For this review, take the finished solid that the model builds, in its own axes (mm). A direction names the side the tool comes from. Give positions to 0.01 mm unless a question says otherwise; leave off trailing zeros. Loops run counter-clockwise (first coordinate to the right, second up) from the corner with the lowest first, then second, coordinate; pieces in that order, holes last. Notation, with made-up numbers: (42, 71.5) - (85, 71.5) arc R14 ccw to (85, 79.5) - close; hole circle Ø10 at (88.5, 31.5). An arc over 180 degrees is marked (long way). Answer in a Markdown table with one row per item.
Autodesk Inventor part; units mm, degrees
ref_plane "YZ Plane" through (0, 0, 0) normal (1, 0, 0) x (0, 1, 0)
ref_plane "XZ Plane" through (0, 0, 0) normal (0, 1, 0) x (-1, 0, 0)
ref_plane "XY Plane" through (0, 0, 0) normal (0, 0, 1) x (1, 0, 0)
sketch "Boceto1" plane through (0, 0, 0) normal (0, 0, 1) x (1, 0, 0)
  line L0 (-17.5, 10) -> (17.5, 10)
  line L1 (17.5, 10) -> (17.5, -10)
  line L2 (17.5, -10) -> (-17.5, -10)
  line L3 (-17.5, -10) -> (-17.5, 10)
  line L4 (0, 0) -> (0, 1.7227)
  line L5 (0, 0) -> (-2.1619, 0)
  line L6 (17.5, -10) -> (-0.5, -10)
  line L7 (-0.5, -10) -> (-0.5, -27)
  line L8 (-0.5, -27) -> (17.5, -27)
  line L9 (17.5, -27) -> (17.5, -10)
  circle A0 centre (12.5, 0) radius 2
  circle A1 centre (-12.5, 0) radius 2
  point P0 (-0.5, -10)
  dimension "d14" = 35
  dimension "d15" = 20
  dimension "d16" = 18
  dimension "d17" = 17
  dimension "d18" = 4
  dimension "d19" = 4
  dimension "d20" = 5
  dimension "d21" = 5
extrude "Extrusión1" add sketch "Boceto1" along normal blind 10
sketch "Boceto2" plane through (-0.5, -27, 0) normal (0, -1, 0) x (1, 0, 0)
  line L0 (18, 10) -> (-17, 10)
  line L1 (18, 10) -> (-2, 10)
  line L2 (-2, 10) -> (-2, -20)
  line L3 (-2, -20) -> (18, -20)
  line L4 (18, -20) -> (18, 10)
  point P0 (0.5, 0)
  point P1 (-2, 10)
  dimension "d22" = 30
  dimension "d53" = 20
extrude "Extrusión2" add sketch "Boceto2" along normal blind 5
sketch "Boceto4" plane through (-17.5, -10, 0) normal (-1, 0, 0) x (0, 0, 1)
  line L0 (0, 0) -> (0, -17)
  line L1 (10, 20) -> (10, 0)
  line L2 (10, 0) -> (-20, 0)
  line L3 (-20, 0) -> (-20, -5)
  line L4 (-20, -5) -> (10, -5)
  line L5 (10, -5) -> (10, 0)
  line L6 (10, -22) -> (-20, -22)
  point P0 (0, 10)
  dimension "d32" = 5
  dimension "d43" = 30
  dimension "d44" = 30
extrude "Extrusión4" add sketch "Boceto4" against normal up to surface (35 mm away)
sketch "Boceto5" plane through (-0.5, -32, 0) normal (0, -1, 0) x (1, 0, 0)
  circle A0 centre (8, -9) radius 1.75
  line L0 (18, -20) -> (18, 10)
  circle A1 centre (-12, -9) radius 1.75
  line L1 (-2, -20) -> (18, -20)
  line L2 (-17, -20) -> (18, -20)
  line L3 (-17, -20) -> (-17, 10)
  line L4 (-17, 0) -> (18, 0)
  point P0 (0.5, 0)
  point P1 (0, 0)
  dimension "d33" = 3.5
  dimension "d34" = 10
  dimension "d37" = 3.5
  dimension "d38" = 5
  dimension "d41" = 9
  dimension "d42" = 9
extrude "Extrusión5" cut sketch "Boceto5" against normal up to surface (22 mm away) contours A0 | A1
sketch "Boceto7" plane through (17.5, -27, -20) normal (0, 0, -1) x (-1, 0, 0)
  line L0 (0, -5) -> (20, -5)
  line L1 (35, 17) -> (0, 17)
  line L2 (10, -5) -> (10, -5.3641)
  line L3 (13.5, -5) -> (13.5, 17)
  line L4 (6.5, -5) -> (6.5, 17)
  point P0 (17.5, 27)
  dimension "d47" = 7
extrude "Extrusión7" add sketch "Boceto7" along normal blind 5
equation "\"d19\" = d18"
equation "\"d20\" = d21"
equation "\"d44\" = d43"
equation "\"d37\" = d33"
properties part number "Soporte Idler Z" material "Hormigón reforzado con fibra de vidrio"
1. We need section D-D, the plane z = -18. Give the boundary of the cut face in (x, y), and give its area (3 significant figures).
Values:
| item | result |
|---|---|
| outline | (-17.5, -15) - (17.5, -15) - (17.5, -10) - (-17.5, -10) - close; (-2.5, -32) - (17.5, -32) - (17.5, -27) - (-2.5, -27) - close |
| area | 275 mm^2 |
2. Mouldability with a two-part tool opening along Z and no side actions: class faces 6 (the face through (-2.5, -29, -5)), 7 (the face through (14, -29, -20)), 8 (the face through (8.4, -29.5, -7.5)) as released by +Z, released by -Z, zero draft, split by the parting line, or undercut.
Values:
| item | result |
|---|---|
| face 6 | zero draft |
| face 7 | released by -Z |
| face 8 | undercut |
3. Clearance check with flat-ended pins moving along their axes: pin 1 (2.5 mm diameter, centred on x = 15.5, y = -29, fed in from -Z); pin 2 (4 mm diameter, centred on y = -25.5, z = -4, fed in from -X); pin 3 (1.5 mm diameter, centred on y = -21, z = -23, fed in from -X); pin 4 (12 mm diameter, centred on y = -6.5, z = -2.5, fed in from +X). State where each tip first meets the part, or that it passes through.
Values:
| item | result |
|---|---|
| pin 1 | stops at z = -20 |
| pin 2 | stops at x = -2.5 |
| pin 3 | stops at x = 4 |
| pin 4 | stops at x = 17.5 |
4. For faces 1 (the face through (8, -21, 0)), 2 (the face through (14, -12, -20)), 3 (the face through (0, 0, 0)), 4 (the face through (-0.5, -21, 5)), 5 (the face through (4, -21, -22)), list the 3-axis set-ups (+Z, -Z, +X, -X, +Y, -Y) from which the entire face can be reached by the end or side of a thin tool; tool diameter is ignored.
Values:
| item | result |
|---|---|
| face 1 | +X, -X |
| face 2 | -Z, +X, +Y, -Y |
| face 3 | -Z, +X, -X, +Y |
| face 4 | +Z, -Z, -X |
| face 5 | -Z, -X, +Y, -Y |
5. We need section C-C, the plane x = -12.5. Give the boundary of the cut face in (y, z), and give its area (4 significant figures).
Values:
| item | result |
|---|---|
| outline | (-15, -20) - (-10, -20) - (-10, -10.75) - (-15, -10.75) - close; (-15, -7.25) - (-10, -7.25) - (-10, 0) - (-2, 0) - (-2, 10) - (-15, 10) - close; (2, 0) - (10, 0) - (10, 10) - (2, 10) - close |
| area | 292.5 mm^2 |
6. We need section B-B, the plane z = 5. Give the boundary of the cut face in (x, y), and give its area (3 significant figures).
Values:
| item | result |
|---|---|
| outline | (-17.5, -15) - (-0.5, -15) - (-0.5, -27) - (-2.5, -27) - (-2.5, -32) - (17.5, -32) - (17.5, 10) - (-17.5, 10) - close; hole circle Ø4 at (-12.5, 0); hole circle Ø4 at (12.5, 0) |
| area | 1,170 mm^2 |
7. Wall thickness on line 1 (Y direction, x = 7.5, z = -18.5); line 2 (Z direction, x = 8.5, y = -24); line 3 (X direction, y = 0.5, z = 4): over which ranges is each line inside the solid? List them lowest first. Write a range as [from, to].
Values:
| item | result |
|---|---|
| line 1 | y = [-32, -27], [-15, -10] |
| line 2 | z = [-25, -20], [0, 10] |
| line 3 | x = [-17.5, -14.44], [-10.56, 10.56], [14.44, 17.5] |
8. We need section A-A, the plane y = 0. Give the boundary of the cut face in (x, z).
Values:
| item | result |
|---|---|
| outline | (-17.5, 0) - (-14.5, 0) - (-14.5, 10) - (-17.5, 10) - close; (-10.5, 0) - (10.5, 0) - (10.5, 10) - (-10.5, 10) - close; (14.5, 0) - (17.5, 0) - (17.5, 10) - (14.5, 10) - close |
